```python
from build123d import *

# Parameters (mm, degrees)
CROQUIS1_W                       = 127
CROQUIS1_H                       = 120
SALIENTE_EXTRUIR1_DEPTH          = 40
CROQUIS2_W                       = 115
CROQUIS2_H                       = 108
CORTAR_EXTRUIR1_DEPTH            = 20
CROQUIS15_W                      = 16
CROQUIS15_H                      = 15
CORTAR_EXTRUIR3_DEPTH            = 14
REDONDEO4_R                      = 1
REDONDEO5_R                      = 1
TALADRO_DE_MARGEN_PARA_M31_D     = 3.2
TALADRO_DE_MARGEN_PARA_M31_DEPTH = 15
TALADRO_DE_MARGEN_PARA_M31_TIP   = 0.96137699
SALIENTE_EXTRUIR4_DEPTH          = 15
CROQUIS22_W                      = 1.5
CROQUIS22_H                      = 21
SALIENTE_EXTRUIR5_DEPTH          = 5
CROQUIS24_W                      = 38.033070537
CROQUIS24_H                      = 33.923090476
CROQUIS24_R                      = 12.5
SALIENTE_EXTRUIR8_DEPTH          = 5
CROQUIS25_W                      = 14
CROQUIS25_H                      = 6.45894104
CORTAR_EXTRUIR4_DEPTH            = 5
CROQUIS27_W                      = 14
CROQUIS27_H                      = 16.815098629
CORTAR_EXTRUIR5_DEPTH            = 84.1
CROQUIS28_W                      = 15
CROQUIS28_H                      = 15
CORTAR_EXTRUIR6_DEPTH            = 10
REDONDEO7_R                      = 1
CROQUIS32_OUTSIDE_W              = 164.85
CROQUIS32_OUTSIDE_H              = 157.85
CROQUIS32_OUTSIDE_W_2            = 123
CROQUIS32_OUTSIDE_H_2            = 116
CORTAR_EXTRUIR7_DEPTH            = 2
CROQUIS34_W                      = 24
CROQUIS34_H                      = 34
CORTAR_EXTRUIR8_DEPTH            = 4
CROQUIS35_W                      = 2
CROQUIS35_H                      = 24
CORTAR_EXTRUIR9_DEPTH            = 20
REDONDEO13_R                     = 1
REDONDEO19_R                     = 1
REDONDEO14_R                     = 1
CROQUIS36_R                      = 2.5
CORTAR_EXTRUIR10_DEPTH           = 1
CORTAR_EXTRUIR14_DEPTH           = 39
CROQUIS45_W                      = 25.554294357
CROQUIS45_H                      = 77.944282849
CORTAR_EXTRUIR15_DEPTH           = 16
CORTAR_EXTRUIR16_DEPTH           = 31


with BuildPart() as part:
    # Croquis1 → Saliente-Extruir1 (new body)
    with BuildSketch(Plane(origin=(0, 0, 0), x_dir=(1, 0, 0), z_dir=(0, 1, 0))):
        with Locations((12.465540006, -22.149251677)):
            Rectangle(CROQUIS1_W, CROQUIS1_H)
    extrude(amount=SALIENTE_EXTRUIR1_DEPTH)

    # Croquis2 → Cortar-Extruir1 (cut)
    with BuildSketch(Plane(origin=(0, 40, 0), x_dir=(1, 0, 0), z_dir=(0, 1, 0))):
        with Locations((12.465540006, -22.149251677)):
            Rectangle(CROQUIS2_W, CROQUIS2_H)
    extrude(amount=-CORTAR_EXTRUIR1_DEPTH, mode=Mode.SUBTRACT)

    # Croquis15 → Cortar-Extruir3 (cut)
    with BuildSketch(Plane(origin=(0, 0, 76.149251677), x_dir=(-1, 0, 0), z_dir=(0, 0, -1))):
        with Locations((27.534459994, 27.5)):
            Rectangle(CROQUIS15_W, CROQUIS15_H)
    extrude(amount=-CORTAR_EXTRUIR3_DEPTH, mode=Mode.SUBTRACT)

    # Redondeo4
    redondeo4_edges = [part.edges().sort_by_distance(p)[0] for p in [
        (-35.534459994, 35, 79.149251677),
        (-35.534459994, 20, 79.149251677),
        (-19.534459994, 20, 79.149251677),
        (-19.534459994, 35, 79.149251677),
    ]]
    fillet(redondeo4_edges, radius=REDONDEO4_R)

    # Redondeo5
    redondeo5_edges = [part.edges().sort_by_distance(p)[0] for p in [
        (-45.034459994, 30, 76.149251677),
        (69.965540006, 30, 76.149251677),
    ]]
    fillet(redondeo5_edges, radius=REDONDEO5_R)

    # Taladro de margen para M31
    with Locations(Plane(origin=(0, 20, 0), x_dir=(1, 0, 0), z_dir=(0, 1, 0))):
        with Locations((-41.034459994, -57.549251677), (6.965509678, -59.149251677), (-25.815009056, -7.199797633), (1.865509678, -7.156454516)):
            Hole(TALADRO_DE_MARGEN_PARA_M31_D / 2, depth=TALADRO_DE_MARGEN_PARA_M31_DEPTH)
            with Locations((0, 0, -(TALADRO_DE_MARGEN_PARA_M31_DEPTH + TALADRO_DE_MARGEN_PARA_M31_TIP / 2))):  # 118° drill point
                Cone(0, TALADRO_DE_MARGEN_PARA_M31_D / 2, TALADRO_DE_MARGEN_PARA_M31_TIP, mode=Mode.SUBTRACT)

    # Croquis21 → Saliente-Extruir4 (add)
    with BuildSketch(Plane(origin=(0, 20, 0), x_dir=(1, 0, 0), z_dir=(0, 1, 0))):
        Polygon((-45.034459994, -2.072342153), (11.965540006, -2.072342153), (11.965540006, 10.850748323), (69.965540006, 10.850748323), (69.965540006, 31.850748323), (-45.034459994, 31.850748323), align=None)
    extrude(amount=SALIENTE_EXTRUIR4_DEPTH)

    # Croquis22 → Saliente-Extruir5 (add)
    with BuildSketch(Plane(origin=(0, 35, 0), x_dir=(1, 0, 0), z_dir=(0, 1, 0))):
        with Locations((54.215540006, 21.350748323)):
            Rectangle(CROQUIS22_W, CROQUIS22_H)
        with Locations((36.715540006, 21.350748323)):
            Rectangle(CROQUIS22_W, CROQUIS22_H)
    extrude(amount=SALIENTE_EXTRUIR5_DEPTH)

    # Croquis24 → Saliente-Extruir8 (add)
    with BuildSketch(Plane(origin=(0, 35, 0), x_dir=(1, 0, 0), z_dir=(0, 1, 0))):
        with Locations((-26.017924726, 14.889203085)):
            Rectangle(CROQUIS24_W, CROQUIS24_H)
        with Locations(Location((-25.871478116, 14.742756476, 0), (0, 0, 270))):
            Circle(CROQUIS24_R, mode=Mode.SUBTRACT)
    extrude(amount=SALIENTE_EXTRUIR8_DEPTH)

    # Croquis25 → Cortar-Extruir4 (cut)
    with BuildSketch(Plane(origin=(0, 40, 0), x_dir=(1, 0, 0), z_dir=(0, 1, 0))):
        with Locations((-25.871478116, 1.157128367)):
            Rectangle(CROQUIS25_W, CROQUIS25_H)
    extrude(amount=-CORTAR_EXTRUIR4_DEPTH, mode=Mode.SUBTRACT)

    # Croquis27 → Cortar-Extruir5 (cut)
    with BuildSketch(Plane(origin=(0, 35, 0), x_dir=(1, 0, 0), z_dir=(0, 1, 0))):
        with Locations((-25.871478116, 6.335207161)):
            Rectangle(CROQUIS27_W, CROQUIS27_H)
    extrude(amount=-CORTAR_EXTRUIR5_DEPTH, mode=Mode.SUBTRACT)

    # Croquis28 → Cortar-Extruir6 (cut)
    with BuildSketch(Plane.XY.offset(82.149251677)):
        with Locations((2.465540006, 27.5)):
            Rectangle(CROQUIS28_W, CROQUIS28_H)
    extrude(amount=-CORTAR_EXTRUIR6_DEPTH, mode=Mode.SUBTRACT)

    # Redondeo7
    redondeo7_edges = [part.edges().sort_by_distance(p)[0] for p in [
        (-5.034459994, 20, 79.149251677),
        (-5.034459994, 35, 79.149251677),
        (9.965540006, 35, 79.149251677),
        (9.965540006, 20, 79.149251677),
    ]]
    fillet(redondeo7_edges, radius=REDONDEO7_R)

    # Croquis32 outside → Cortar-Extruir7 (cut)
    with BuildSketch(Plane(origin=(0, 40, 0), x_dir=(1, 0, 0), z_dir=(0, 1, 0))):
        with Locations((12.466, -22.149)):
            Rectangle(CROQUIS32_OUTSIDE_W, CROQUIS32_OUTSIDE_H)
        with Locations((12.465540006, -22.149251677)):
            Rectangle(CROQUIS32_OUTSIDE_W_2, CROQUIS32_OUTSIDE_H_2, mode=Mode.SUBTRACT)
    extrude(amount=-CORTAR_EXTRUIR7_DEPTH, mode=Mode.SUBTRACT)

    # Croquis34 → Cortar-Extruir8 (cut)
    with BuildSketch(Plane(origin=(75.965540006, 0, 0), x_dir=(0, 0, -1), z_dir=(1, 0, 0))):
        with Locations((-48.149251677, 17)):
            Rectangle(CROQUIS34_W, CROQUIS34_H)
        with Locations((3.850748323, 17)):
            Rectangle(CROQUIS34_W, CROQUIS34_H)
    cortar_extruir8 = extrude(amount=-CORTAR_EXTRUIR8_DEPTH, mode=Mode.SUBTRACT)

    # Croquis35 → Cortar-Extruir9 (cut)
    with BuildSketch(Plane.XZ.offset(-34)):
        with Locations((72.965540006, 48.149251677)):
            Rectangle(CROQUIS35_W, CROQUIS35_H)
        with Locations((72.965540006, -3.850748323)):
            Rectangle(CROQUIS35_W, CROQUIS35_H)
    cortar_extruir9 = extrude(amount=-CORTAR_EXTRUIR9_DEPTH, mode=Mode.SUBTRACT)

    # Redondeo13
    redondeo13_edges = [part.edges().sort_by_distance(p)[0] for p in [
        (71.965540006, 20, 60.149251677),
        (71.965540006, 20, 36.149251677),
        (75.965540006, 17, 60.149251677),
        (75.965540006, 17, 36.149251677),
        (71.965540006, 20, 8.149251677),
        (71.965540006, 20, -15.850748323),
        (75.965540006, 17, 8.149251677),
        (75.965540006, 17, -15.850748323),
    ]]
    fillet(redondeo13_edges, radius=REDONDEO13_R)

    # Simetría2: Cortar-Extruir8, Cortar-Extruir9 across plane
    add(cortar_extruir8.mirror(Plane(origin=(12.465540006, 0, 0), x_dir=(0, 0, 1), z_dir=(1, 0, 0))), mode=Mode.SUBTRACT)
    add(cortar_extruir9.mirror(Plane(origin=(12.465540006, 0, 0), x_dir=(0, 0, 1), z_dir=(1, 0, 0))), mode=Mode.SUBTRACT)

    # Redondeo19
    redondeo19_edges = [part.edges().sort_by_distance(p)[0] for p in [
        (-51.034459994, 17, 60.149251677),
        (-51.034459994, 17, 36.149251677),
        (-51.034459994, 17, 8.149251677),
        (-51.034459994, 17, -15.850748323),
        (-47.034459994, 20, 8.149251677),
        (-47.034459994, 20, -15.850748323),
    ]]
    fillet(redondeo19_edges, radius=REDONDEO19_R)

    # Redondeo14
    redondeo14_edges = [part.edges().sort_by_distance(p)[0] for p in [
        (-51.034459994, 19, 82.149251677),
        (-51.034459994, 19, -37.850748323),
        (75.965540006, 19, -37.850748323),
        (75.965540006, 19, 82.149251677),
    ]]
    fillet(redondeo14_edges, radius=REDONDEO14_R)

    # Croquis36 → Cortar-Extruir10 (cut)
    with BuildSketch(Plane(origin=(0, 0, 0), x_dir=(-1, 0, 0), z_dir=(0, -1, 0))):
        with Locations(Location((-12.465540006, -58.149251677, 0), (0, 0, 90))):
            Circle(CROQUIS36_R)
        with Locations(Location((-12.465540006, 13.850748323, 0), (0, 0, 90))):
            Circle(CROQUIS36_R)
        with Locations(Location((-12.465540006, -10.149251677, 0), (0, 0, 90))):
            Circle(CROQUIS36_R)
        with Locations(Location((-12.465540006, -34.149251677, 0), (0, 0, 90))):
            Circle(CROQUIS36_R)
    extrude(amount=-CORTAR_EXTRUIR10_DEPTH, mode=Mode.SUBTRACT)

    # Croquis44 → Cortar-Extruir14 (cut)
    with BuildSketch(Plane(origin=(0, 35, 0), x_dir=(1, 0, 0), z_dir=(0, 1, 0))):
        with BuildLine():
            Line((49.133290382, 26.728304647), (49.133290382, 15.518377593))
            ThreePointArc((49.133290382, 15.518377593), (45.465540006, 11.850627217), (41.797789631, 15.518377593))
            Line((41.797789631, 15.518377593), (41.797789631, 26.728304647))
            ThreePointArc((41.797789631, 26.728304647), (45.465540006, 30.396055022), (49.133290382, 26.728304647))
        make_face()
        with BuildLine():
            Line((65.633290382, 26.728304647), (65.633290382, 15.518377593))
            ThreePointArc((65.633290382, 15.518377593), (62.465540006, 12.350627217), (59.297789631, 15.518377593))
            Line((59.297789631, 15.518377593), (59.297789631, 26.728304647))
            ThreePointArc((59.297789631, 26.728304647), (62.465540006, 29.896055022), (65.633290382, 26.728304647))
        make_face()
    extrude(amount=-CORTAR_EXTRUIR14_DEPTH, mode=Mode.SUBTRACT)

    # Croquis45 → Cortar-Extruir15 (cut)
    with BuildSketch(Plane(origin=(0, 20, 0), x_dir=(1, 0, 0), z_dir=(0, 1, 0))):
        Polygon((-31.458080568, -4.711128446), (-31.458080568, -11.448349249), (-20.361481599, -11.448349249), (-20.361481599, -4.711128446), (-3.980787883, -4.711128446), (-3.980787883, -11.448349249), (8.040527667, -11.448349249), (8.040527667, -4.711128446), (16.230874525, -4.711128446), (16.230874525, 5.427258738), (33.668387191, 5.427258738), (33.668387191, -72.517024111), (13.808026092, -72.517024111), (13.808026092, -52.728826942), (0, -52.728826942), (0, -72.517024111), (-36.514276642, -72.517024111), (-36.514276642, -51.287302645), (-41.88723084, -51.287302645), (-41.88723084, -4.711128446), align=None)
        with Locations((51.091086321, -33.544882686)):
            Rectangle(CROQUIS45_W, CROQUIS45_H)
    extrude(amount=-CORTAR_EXTRUIR15_DEPTH, mode=Mode.SUBTRACT)

    # Croquis46 → Cortar-Extruir16 (cut)
    with BuildSketch(Plane(origin=(0, 35, 0), x_dir=(1, 0, 0), z_dir=(0, 1, 0))):
        Polygon((-7.001389457, 31.850748323), (35.965540006, 31.850748323), (35.965540006, 10.850748323), (11.965540006, 10.850748323), (11.965540006, -2.072342153), (-7.001389457, -2.072342153), align=None)
    extrude(amount=-CORTAR_EXTRUIR16_DEPTH, mode=Mode.SUBTRACT)


solid = part.part
```
Build history of the part. All positions in model axes, mm. A direction names the side the tool comes from. Coordinates: 2 decimals unless noted, no trailing zeros. Order: outer loops, then holes, each group sorted by start corner. A loop starts at its lowest first (then second) coordinate and runs counter-clockwise, first axis right, second up.
Item 1: Saw through at C-C on x = 62. List the corners of the cut face in (y, z).
Filled in:
outline: (0, -37.85) - (38, -37.85) - (38, -35.85) - (40, -35.85) - (40, -31.85) - (35, -31.85) - (35, -29.86) - (0, -29.86) - close; (0, -12.39) - (35, -12.39) - (35, -10.85) - (20, -10.85) - (20, -5.43) - (4, -5.43) - (4, 72.52) - (20, 72.52) - (20, 76.15) - (40, 76.15) - (40, 80.15) - (38, 80.15) - (38, 82.15) - (0, 82.15) - close
Item 2: Tool access for faces 1 (the flat face through (12, 12, 4.711)), 2 (the flat face through (-26, 10, 2.072)), 3 (the flat face through (9.966, 27, 79)), 4 (the flat face through (13, 1, 58)): list every direction of +Z, -Z, +X, -X, +Y, -Y with a clear straight run to the whole face (end or side of a thin tool).
Filled in:
face 1: +Y
face 2: +Y, -Y
face 3: +Z
face 4: -Y
Item 3: Saw through at D-D on z = 65. List the corners of the cut face in (x, y).
Filled in:
outline: (-51.03, 0) - (75.97, 0) - (75.97, 38) - (73.97, 38) - (73.97, 40) - (69.97, 40) - (69.97, 20) - (63.87, 20) - (63.87, 4) - (38.31, 4) - (38.31, 20) - (33.67, 20) - (33.67, 4) - (13.81, 4) - (13.81, 20) - (0, 20) - (0, 4) - (-36.51, 4) - (-36.51, 20) - (-45.03, 20) - (-45.03, 40) - (-49.03, 40) - (-49.03, 38) - (-51.03, 38) - close
Item 4: Saw through at A-A on z = 41.5. List the corners of the cut face in (x, y).
Filled in:
outline: (-51.03, 34) - (-49.03, 34) - (-49.03, 38) - (-51.03, 38) - close; (-47.03, 0) - (71.97, 0) - (71.97, 40) - (69.97, 40) - (69.97, 20) - (63.87, 20) - (63.87, 4) - (38.31, 4) - (38.31, 20) - (33.67, 20) - (33.67, 4) - (-41.89, 4) - (-41.89, 20) - (-45.03, 20) - (-45.03, 40) - (-47.03, 40) - close; (73.97, 34) - (75.97, 34) - (75.97, 38) - (73.97, 38) - close
Item 5: Saw through at B-B on y = 29.5. State how many separate pieces and enclosed holes the cut face has, then the cut area to 3 significant figures.
Filled in:
separate pieces: 2
enclosed holes: 2
area: 3,790 mm2
Item 6: Drop flat-ended pins along their axis: pin 1 Ø20 at (x, z) = (-25.87, -14.74) entering from +Y; pin 2 Ø0.6 at (y, z) = (39, 65.5) entering from +X; pin 3 Ø4.5 at (x, z) = (12.47, 58.15) entering from -Y. Give the stop position or say it passes through.
Filled in:
pin 1: stops at y = 35
pin 2: stops at x = 73.97
pin 3: stops at y = 1
Item 7: Drill centre lines: L1, parallel to X at y = 6, z = 2.5; L2, parallel to X at y = 8, z = 63; L3, parallel to X at y = 34.5, z = -18. Where is each one in solid material? Low to high.
Filled in:
L1: x = -47.03 to 16.23, 33.67 to 38.31, 63.87 to 71.97
L2: x = -51.03 to -36.51, 0 to 13.81, 33.67 to 38.31, 63.87 to 75.97
L3: x = -51.03 to -7, 35.97 to 41.8, 49.13 to 59.3, 65.63 to 75.97
